Read the model definition and answer for the solid it produces. Units are mm, in the model's axes. Face numbers are marked on the shaded views. A direction names the side the tool comes from. Round coordinates to 2 decimals unless told otherwise and drop trailing zeros. Order: outer loops, then holes, each group sorted by start corner. A loop starts at its lowest first (then second) coordinate and runs counter-clockwise, first axis right, second up. Notation, with made-up numbers: (18.5, -7) -> (24.5, -7) arc R11 cw to (24.5, 6) -> close; hole circle Ø11 at (-24, 44.5). An arc over 180 degrees is marked (long way). One line per item, written item: value. Start each with the question number.
1. Consider line 1 (X direction, y = -1.25, z = 4.75); line 2 (X direction, y = -0.5, z = 10); line 3 (Y direction, x = -0.25, z = 6.25). Determine where each line is inside the solid, lowest interval first.
2. Section A-A (z = 4) is taken. Give the vertices of the cut face in (x, y).
3. Flat-ended cylindrical pins translate along their axes: pin 1 Ø1.5 at (x, z) = (0.5, 8.5) entering from +Y; pin 2 Ø1.5 at (y, z) = (-2, 9) entering from -X; pin 3 Ø1 at (y, z) = (1.5, 6) entering from -X. Find the tip coordinate at first contact, or state that the pin passes through.
4. For the marked faces 1 and 2, determine the directions among +Z, -Z, +X, -X, +Y, -Y from which every point of the face is accessible in a straight line to the end or side of a thin tool.
Autodesk Inventor part; units mm, degrees
ref_plane "YZ Plane" through (0, 0, 0) normal (1, 0, 0) x (0, 1, 0)
ref_plane "XZ Plane" through (0, 0, 0) normal (0, 1, 0) x (-1, 0, 0)
ref_plane "XY Plane" through (0, 0, 0) normal (0, 0, 1) x (1, 0, 0)
sketch "スケッチ1" plane through (0, 0, 0) normal (0, 0, 1) x (1, 0, 0)
  circle A0 centre (0, 0) radius 1.5
  dimension "d0" = 3
extrude "押し出し1" add sketch "スケッチ1" along normal blind 12
sketch "スケッチ2" plane through (0, 0, 12) normal (0, 0, 1) x (1, 0, 0)
  circle A0 centre (0, 0) radius 1.5
  circle A1 centre (0, 0) radius 3
  dimension "d3" = 6
extrude "押し出し2" add sketch "スケッチ2" along normal blind 2 contours A0 | A1
fillet "フィレット1" radius 2 1 edges at (-3, 0, 14)
properties part number "M3ボタンボルト12" material "鋼、高強度、低合金"
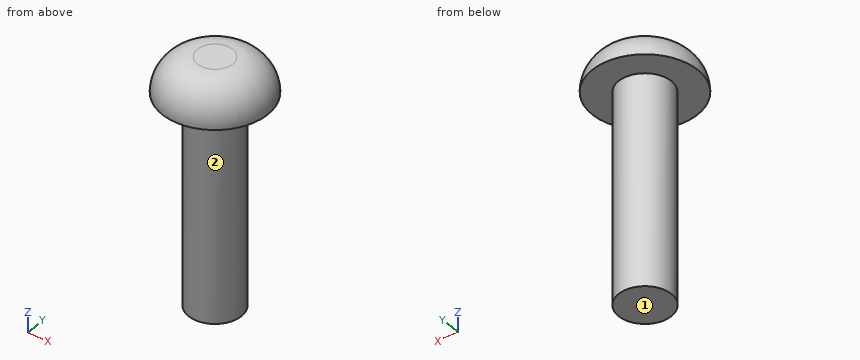
Answer:
1. line 1: -0.83 to 0.83
1. line 2: -1.41 to 1.41
1. line 3: -1.48 to 1.48
2. outline: circle Ø3 at (0, 0)
3. pin 1: y = 1.5
3. pin 2: x = -0.83
3. pin 3: x = -1.12
4. face 1: -Z, +X, -X, +Y, -Y
4. face 2: -Z
